from build123d import *

# Parameters (mm, degrees)
F0_R     = 3
F1_DEPTH = 14


with BuildPart() as f1:
    # F0 (on Front) → F1 (new body)
    with BuildSketch(Plane.XZ):
        with BuildLine():
            ThreePointArc((-16.492189, 19.927121), (-24.474129, 11.389875), (-15.420123, 3.999279))
            Line((-15.420123, 3.999279), (15.717345, 3.999279))
            ThreePointArc((15.717345, 3.999279), (23.454399, 12.041669), (15.521441, 19.890888))
            Line((15.521441, 19.890888), (15.521441, 27.943708))
            Line((15.521441, 27.943708), (-4.478559, 27.943708))
            Line((-4.478559, 27.943708), (-4.478559, 19.927121))
            Line((-4.478559, 19.927121), (-16.492189, 19.927121))
        make_face()
        with Locations((-16.492189, 11.927121)):
            Circle(F0_R, mode=Mode.SUBTRACT)
        with Locations((15.507811, 11.943708)):
            Circle(F0_R, mode=Mode.SUBTRACT)
    extrude(amount=-F1_DEPTH)


solid = f1.part
Read the model definition and answer for the solid it produces. Units are mm, in the model's axes. A direction names the side the tool comes from. Coordinates: 2 decimals unless noted, no trailing zeros. Order: outer loops, then holes, each group sorted by start corner. A loop starts at its lowest first (then second) coordinate and runs counter-clockwise, first axis right, second up. Notation, with made-up numbers: (12, -40) -> (58, -40) arc R25 cw to (58, -3) -> close; hole circle Ø4 at (6.25, 44.25). An arc over 180 degrees is marked (long way). Answer as a JSON object with one key per item and string values.
1) A tool of negligible diameter and unlimited length cuts with its end or side. For faces 1 (the face through (15.521, 7, 24)), 2 (the face through (-4.479, 7, 24)), 3 (the face through (17.121, 6.902, 14.473)), 4 (the face through (6, 7, 27.944)), 5 (the face through (0, 7, 3.999)), from which of +Z, -Z, +X, -X, +Y, -Y can it reach the whole face along a straight path? Write none if from no direction.
Model answer:
{"face 1": "+Z, +X, +Y, -Y", "face 2": "+Z, -X, +Y, -Y", "face 3": "+Y, -Y", "face 4": "+Z, +X, -X, +Y, -Y", "face 5": "-Z, +X, +Y, -Y"}
2) A cutting plane is placed at C-C, the plane y = 10.5. Determine the outline of the cut face in (x, z).
Model answer:
{"outline": "(-16.49, 19.93) arc R8 ccw (long way) to (-15.42, 4) -> (15.72, 4) arc R7.95 ccw to (15.52, 19.89) -> (15.52, 27.94) -> (-4.48, 27.94) -> (-4.48, 19.93) -> close; hole circle Ø6 at (-16.49, 11.93); hole circle Ø6 at (15.51, 11.94)"}
3) The mould has two halves that part along Z. Classify faces 6 (the face through (-18.703, 6.902, 13.955)), 7 (the face through (23.455, 6.902, 11.868)), 8 (the face through (-1, 0, 13)): released by +Z, released by -Z, zero draft, split by the parting line, or undercut.
Model answer:
{"face 6": "undercut", "face 7": "split by the parting line", "face 8": "zero draft"}
4) Consider line 1 along X through (y, z) = (11.5, 13.5); line 2 along X through (y, z) = (1, 10.25); line 3 along X through (y, z) = (2, 22.25). Determine where each line is inside the solid, lowest interval first. Write a range as from..to.
Model answer:
{"line 1": "x = -24.34..-19.05, -13.94..12.94, 18.07..23.3", "line 2": "x = -24.31..-18.98, -14..13.03, 17.98..23.27", "line 3": "x = -4.48..15.52"}
5) A cutting plane is placed at A-A, the plane z = 10.5. Determine the outline of the cut face in (x, y).
Model answer:
{"outline": "(-24.36, 0) -> (-19.13, 0) -> (-19.13, 14) -> (-24.36, 14) -> close; (-13.85, 0) -> (12.88, 0) -> (12.88, 14) -> (-13.85, 14) -> close; (18.14, 0) -> (23.32, 0) -> (23.32, 14) -> (18.14, 14) -> close"}
6) Each of these flat-tipped pins is pushed along its axis until it touches: pin 1 (2 mm diameter, centred on y = 10, z = 15.5, fed in from +X); pin 2 (4 mm diameter, centred on y = 9.5, z = 25.5, fed in from -X); pin 3 (1.5 mm diameter, centred on x = 11, y = 9, fed in from -Z); pin 4 (3.5 mm diameter, centred on x = -16.49, z = 11.93, fed in from -Y). Where does it stop, or does it pass through?
Model answer:
{"pin 1": "stops at x = 23.03", "pin 2": "stops at x = -4.48", "pin 3": "stops at z = 4", "pin 4": "passes through"}
7) A cutting plane is placed at B-B, the plane x = 17. Determine the outline of the cut face in (y, z), plus the area to 3 significant figures.
Model answer:
{"outline": "(0, 4.14) -> (14, 4.14) -> (14, 9.34) -> (0, 9.34) -> close; (0, 14.55) -> (14, 14.55) -> (14, 19.75) -> (0, 19.75) -> close", "area": "146 mm²"}
8) A cutting plane is placed at D-D, the plane x = -10.5. Determine the outline of the cut face in (y, z).
Model answer:
{"outline": "(0, 4) -> (14, 4) -> (14, 19.93) -> (0, 19.93) -> close"}
